Verification items for the finished model (mm, model axes). Face numbers are marked on the shaded views. A direction names the side the tool comes from. Give positions to 0.01 mm unless a question says otherwise; leave off trailing zeros. Order: outer loops, then holes, each group sorted by start corner. A loop starts at its lowest first (then second) coordinate and runs counter-clockwise, first axis right, second up. Notation, with made-up numbers: (6.5, -15) - (23.5, -15) arc R30 cw to (23.5, 14) - close; hole circle Ø3 at (63, 82.25). An arc over 180 degrees is marked (long way). Answer as a JSON object with one key per item and string values.
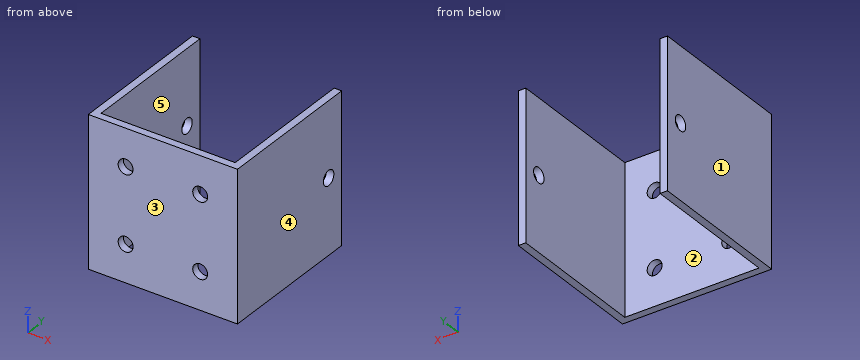
Autodesk Inventor part; units mm, degrees
ref_plane "YZ Plane" through (0, 0, 0) normal (1, 0, 0) x (0, 1, 0)
ref_plane "XZ Plane" through (0, 0, 0) normal (0, 1, 0) x (-1, 0, 0)
ref_plane "XY Plane" through (0, 0, 0) normal (0, 0, 1) x (1, 0, 0)
sketch "スケッチ1" plane through (0, 0, 0) normal (0, 1, 0) x (-1, 0, 0)
  line L0 (20, 20) -> (-20, 20)
  line L1 (-20, 20) -> (-20, -20)
  line L2 (-20, -20) -> (20, -20)
  line L3 (20, -20) -> (20, 20)
  line L4 (20, 20) -> (-20, -20) construction
  line L5 (-20, 20) -> (20, -20) construction
  point P0 (0, 0)
  dimension "d0" = 40
  dimension "d1" = 40
extrude "押し出し1" add sketch "スケッチ1" along normal blind 40
sketch "スケッチ2" plane through (0, 40, 0) normal (0, 1, 0) x (1, 0, 0)
  line L0 (20, 20) -> (-20, 20)
  line L1 (-18, -20) -> (18, -20)
  line L2 (18, -20) -> (18, 20)
  line L3 (18, 20) -> (-18, 20)
  line L4 (-18, 20) -> (-18, -20)
  line L5 (-18, -20) -> (18, 20) construction
  line L6 (18, -20) -> (-18, 20) construction
  point P0 (0, 0)
  dimension "d4" = 36
extrude "押し出し2" cut sketch "スケッチ2" against normal blind 38
sketch "スケッチ3" plane through (0, 0, 0) normal (0, -1, 0) x (1, 0, 0)
  line L0 (-20, 20) -> (20, 20)
  line L1 (20, 20) -> (20, -20)
  point P0 (0, 0)
  point P1 (10, 10)
  point P2 (10, -10)
  point P3 (-10, 10)
  point P4 (-10, -10)
  dimension "d7" = 10
  dimension "d8" = 10
  dimension "d11" = 20
  dimension "d14" = 20
hole "穴1" at (10, 0, 10) at (10, 0, -10) at (-10, 0, 10) at (-10, 0, -10) direction (0, 1, 0) diameter 4 end through all
sketch "スケッチ4" plane through (20, 0, 20) normal (1, 0, 0) x (0, 0, -1)
  line L0 (0, 40) -> (40, 40)
  line L1 (0, 0) -> (0, 40)
  point P0 (20, 0)
  point P1 (20, 35)
  dimension "d24" = 5
  dimension "d25" = 20
hole "穴2" at (20, 35, 0) direction (-1, 0, 0) diameter 4 end through all
properties part number "blaket_1"
(1) Section check B-B (z = -10). Record the cut outline in (x, y), then the cut area to 3 significant figures.
Computed values:
{"outline": "(-20, 0) - (-12, 0) - (-12, 2) - (-18, 2) - (-18, 40) - (-20, 40) - close; (-8, 0) - (8, 0) - (8, 2) - (-8, 2) - close; (12, 0) - (20, 0) - (20, 40) - (18, 40) - (18, 2) - (12, 2) - close", "area": "216 mm²"}
(2) Access from +Z, -Z, +X, -X, +Y, -Y to the whole of each face (thin tool, end or side, straight path). Record for the marked faces 1 and 2.
Computed values:
{"face 1": "+Z, -Z, -X, +Y, -Y", "face 2": "+Z, -Z, +Y"}
(3) Section check C-C (x = -10). Record the cut outline in (y, z), then the cut area to 3 significant figures.
Computed values:
{"outline": "(0, -20) - (2, -20) - (2, -12) - (0, -12) - close; (0, -8) - (2, -8) - (2, 8) - (0, 8) - close; (0, 12) - (2, 12) - (2, 20) - (0, 20) - close", "area": "64.0 mm²"}
(4) Release check for a two-part mould opening along X. For the marked faces 3, 4 and 5 record: pulls with the +X half, pulls with the -X half, needs draft (parallel to the pull), parting line crosses it, or undercut.
Computed values:
{"face 3": "needs draft", "face 4": "pulls with the +X half", "face 5": "undercut"}
(5) Section check A-A (y = 22.5). Record the cut outline in (x, z).
Computed values:
{"outline": "(-20, -20) - (-18, -20) - (-18, 20) - (-20, 20) - close; (18, -20) - (20, -20) - (20, 20) - (18, 20) - close"}
(6) Material ranges on line 1 along X through (y, z) = (1, -10); line 2 along X through (y, z) = (4, 8), recorded low to high. Write a range as [from, to].
Computed values:
{"line 1": "x = [-20, -12], [-8, 8], [12, 20]", "line 2": "x = [-20, -18], [18, 20]"}
(7) Gauge pin test, flat ends, axial feed: pin 1 Ø4 at (x, z) = (-6.5, 14.5) entering from +Y; pin 2 Ø3 at (x, z) = (10, 10) entering from -Y; pin 3 Ø5 at (x, z) = (-4, -2.5) entering from -Y. Record the tip position at first contact, or that the pin passes through.
Computed values:
{"pin 1": "stops at y = 2", "pin 2": "passes through", "pin 3": "stops at y = 0"}
(8) Section check D-D (y = 35). Record the cut outline in (x, z).
Computed values:
{"outline": "(-20, -20) - (-18, -20) - (-18, -2) - (-20, -2) - close; (-20, 2) - (-18, 2) - (-18, 20) - (-20, 20) - close; (18, -20) - (20, -20) - (20, -2) - (18, -2) - close; (18, 2) - (20, 2) - (20, 20) - (18, 20) - close"}
